Work out the finished part from the listing and answer in its coordinate system (mm). Face numbers are marked on the shaded views. A direction names the side the tool comes from. Round coordinates to 2 decimals unless told otherwise and drop trailing zeros. Loops run counter-clockwise (first coordinate to the right, second up) from the corner with the lowest first, then second, coordinate; pieces in that order, holes last. Notation, with made-up numbers: (51.5, -28) -> (110.5, -28) arc R17 cw to (110.5, -17) -> close; hole circle Ø10 at (1.25, 65.5). An arc over 180 degrees is marked (long way). Write item = value, one per line. Start each with the question number.
```python
from build123d import *

# Parameters (mm, degrees)
F0_R     = 43.18
F1_DEPTH = 147.32
F2_DEPTH = 104.14
F3_DEPTH = 43.18


with BuildPart() as f1:
    # F0 (on Top) → F1 (new body)
    with BuildSketch(Plane.XY):
        with BuildLine():
            Line((-114.3, 82.55), (-114.3, -82.55))
            Line((-114.3, -82.55), (114.3, -82.55))
            Line((114.3, -82.55), (114.3, 82.55))
            Line((114.3, 82.55), (33.02, 82.55))
            Line((33.02, 82.55), (33.02, 38.099274))
            ThreePointArc((33.02, 38.099274), (52.570446, -23.739841), (0, -61.722))
            ThreePointArc((0, -61.722), (-52.570446, -23.739841), (-33.02, 38.099274))
            Line((-33.02, 38.099274), (-33.02, 82.55))
            Line((-33.02, 82.55), (-114.3, 82.55))
        make_face()
        with BuildLine():
            Line((0, 82.55), (-33.02, 82.55))
            Line((-33.02, 82.55), (-33.02, 38.099274))
            ThreePointArc((-33.02, 38.099274), (-52.570446, -23.739841), (0, -61.722))
            ThreePointArc((0, -61.722), (52.570446, -23.739841), (33.02, 38.099274))
            Line((33.02, 38.099274), (33.02, 82.55))
            Line((33.02, 82.55), (0, 82.55))
        make_face()
        with Locations((0, -6.35)):
            Circle(F0_R, mode=Mode.SUBTRACT)
    extrude(amount=F1_DEPTH)

    # F0 (on Top) → F2 (cut)
    with BuildSketch(Plane.XY):
        with BuildLine():
            Line((-114.3, 82.55), (-114.3, -82.55))
            Line((-114.3, -82.55), (114.3, -82.55))
            Line((114.3, -82.55), (114.3, 82.55))
            Line((114.3, 82.55), (33.02, 82.55))
            Line((33.02, 82.55), (33.02, 38.099274))
            ThreePointArc((33.02, 38.099274), (52.570446, -23.739841), (0, -61.722))
            ThreePointArc((0, -61.722), (-52.570446, -23.739841), (-33.02, 38.099274))
            Line((-33.02, 38.099274), (-33.02, 82.55))
            Line((-33.02, 82.55), (-114.3, 82.55))
        make_face()
    extrude(amount=F2_DEPTH, mode=Mode.SUBTRACT)

    # F0 (on Top) → F3 (join)
    with BuildSketch(Plane.XY):
        with BuildLine():
            Line((-114.3, 82.55), (-114.3, -82.55))
            Line((-114.3, -82.55), (114.3, -82.55))
            Line((114.3, -82.55), (114.3, 82.55))
            Line((114.3, 82.55), (33.02, 82.55))
            Line((33.02, 82.55), (33.02, 38.099274))
            ThreePointArc((33.02, 38.099274), (52.570446, -23.739841), (0, -61.722))
            ThreePointArc((0, -61.722), (-52.570446, -23.739841), (-33.02, 38.099274))
            Line((-33.02, 38.099274), (-33.02, 82.55))
            Line((-33.02, 82.55), (-114.3, 82.55))
        make_face()
    extrude(amount=F3_DEPTH)


solid = f1.part
```
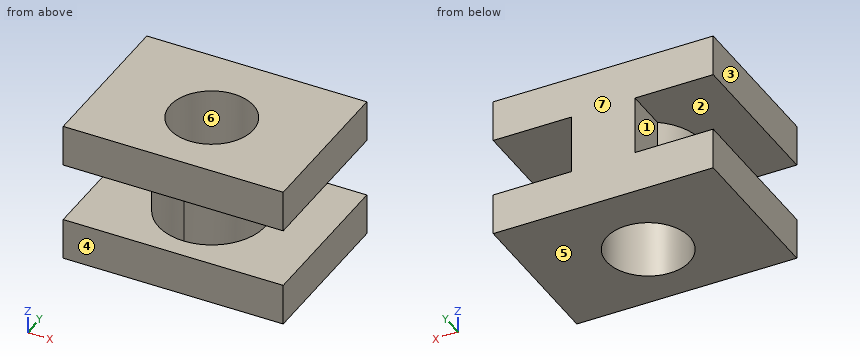
Item 1: Section C-C (z = 119) is taken. Determine the outline of the cut face in (x, y), then the cut area to 3 significant figures.
Item 2: Flat-ended cylindrical pins translate along their axes: pin 1 (13.5 mm diameter, centred on y = 66, z = 73, fed in from +X); pin 2 (13.5 mm diameter, centred on y = 63.5, z = 88, fed in from -X); pin 3 (3 mm diameter, centred on y = -33.5, z = 81.5, fed in from -X). Find the tip coordinate at first contact, or state that the pin passes through.
Item 3: Section D-D (y = 64.5) is taken. Determine the outline of the cut face in (x, z), then the cut area to 3 significant figures.
Item 4: The mould has two halves that part along Y. Classify the marked faces 4, 5, 6 and 7: pulls with the +Y half, pulls with the -Y half, needs draft (parallel to the pull), parting line crosses it, or undercut.
Item 5: A tool of negligible diameter and unlimited length cuts with its end or side. For the marked faces 1, 2 and 3, from which of +Z, -Z, +X, -X, +Y, -Y can it reach the whole face along a straight path? Write none if from no direction.
Item 6: Section A-A (x = 86.5) is taken. Determine the outline of the cut face in (y, z).
Item 7: Find the intervals of material crossed by line 1 along X through (y, z) = (-6, 110); line 2 along X through (y, z) = (-6, 61); line 3 along Z through (x, y) = (-68, -30.5), in increasing order. Write a range as [from, to].
Item 8: Section B-B (y = -6.35) is taken. Determine the outline of the cut face in (x, z).
Worked answers:
q1.outline = (-114.3, -82.55) -> (114.3, -82.55) -> (114.3, 82.55) -> (-114.3, 82.55) -> close; hole circle Ø86.36 at (0, -6.35)
q1.area = 31,900 mm2
q2.pin_1 = 33.02
q2.pin_2 = -33.02
q2.pin_3 = -49.07
q3.outline = (-114.3, 0) -> (114.3, 0) -> (114.3, 43.18) -> (33.02, 43.18) -> (33.02, 104.14) -> (114.3, 104.14) -> (114.3, 147.32) -> (-114.3, 147.32) -> (-114.3, 104.14) -> (-33.02, 104.14) -> (-33.02, 43.18) -> (-114.3, 43.18) -> close
q3.area = 23,800 mm2
q4.face_4 = pulls with the -Y half
q4.face_5 = needs draft
q4.face_6 = undercut
q4.face_7 = pulls with the +Y half
q5.face_1 = -X, +Y
q5.face_2 = none
q5.face_3 = +Z, -Z, -X, +Y, -Y
q6.outline = (-82.55, 0) -> (82.55, 0) -> (82.55, 43.18) -> (-82.55, 43.18) -> close; (-82.55, 104.14) -> (82.55, 104.14) -> (82.55, 147.32) -> (-82.55, 147.32) -> close
q7.line_1 = [-114.3, -43.18], [43.18, 114.3]
q7.line_2 = [-55.37, -43.18], [43.18, 55.37]
q7.line_3 = [0, 43.18], [104.14, 147.32]
q8.outline = (-114.3, 0) -> (-43.18, 0) -> (-43.18, 147.32) -> (-114.3, 147.32) -> (-114.3, 104.14) -> (-55.37, 104.14) -> (-55.37, 43.18) -> (-114.3, 43.18) -> close; (43.18, 0) -> (114.3, 0) -> (114.3, 43.18) -> (55.37, 43.18) -> (55.37, 104.14) -> (114.3, 104.14) -> (114.3, 147.32) -> (43.18, 147.32) -> close
